Here's the drawing with two shaded views (mm, measured from the low corner). I have some questions. A direction names the side the tool comes from. Coordinates: 2 decimals unless noted, no trailing zeros. Order: outer loops, then holes, each group sorted by start corner. A loop starts at its lowest first (then second) coordinate and runs counter-clockwise, first axis right, second up. Notation, with made-up numbers: (-21, -29.75) - (-4, -29.75) arc R31 ccw to (-4, 5.25) - close; hole circle Ø5 at (-34, 13.25). An arc over 180 degrees is marked (long way). Answer as a JSON object with one key per item and string values. Group by question number.
(1) Imagine slicing it at D-D, the plane z = 10. Write out the boundary of the cut face in (x, y) (3 decimals), and give its area (3 significant figures).
(2) Will these pins go through, and if not, where does the flat tip stop? P1, Ø4, axis at x = 22, z = 3.5, coming from the -Y side; P2, Ø1, axis at y = 6, z = 2, coming from the -X side; P3, Ø1, axis at x = 29, z = 3, coming from the +Y side.
(3) Please list where these lines run through material, in increasing order: probe 1 along Y at (x, z) = (4, 3.5) (3 decimals); probe 2 along Z at (x, y) = (17.5, 2); probe 3 along X at (y, z) = (2.5, 9.25).
(4) We'd pull the mould along Y, two halves only. Please class the marked faces 1, 2, 3 and 4: pulls with the +Y half, pulls with the -Y half, needs draft (parallel to the pull), parting line crosses it, or undercut.
(5) Imagine slicing it at A-A, the plane x = 4. Write out the boundary of the cut face in (y, z) (3 decimals), and give its area (3 significant figures).
(6) Imagine slicing it at B-B, the plane y = 3. Write out the boundary of the cut face in (x, z).
(7) Imagine slicing it at C-C, the plane z = 2. Write out the boundary of the cut face in (x, y) (1 decimal), and give its area (3 significant figures).
(8) Which directions (+Z, -Z, +X, -X, +Y, -Y) give clear straight access to the entire face, cutting with the end or side of a thin tool? Please do the marked faces 5 and 6.
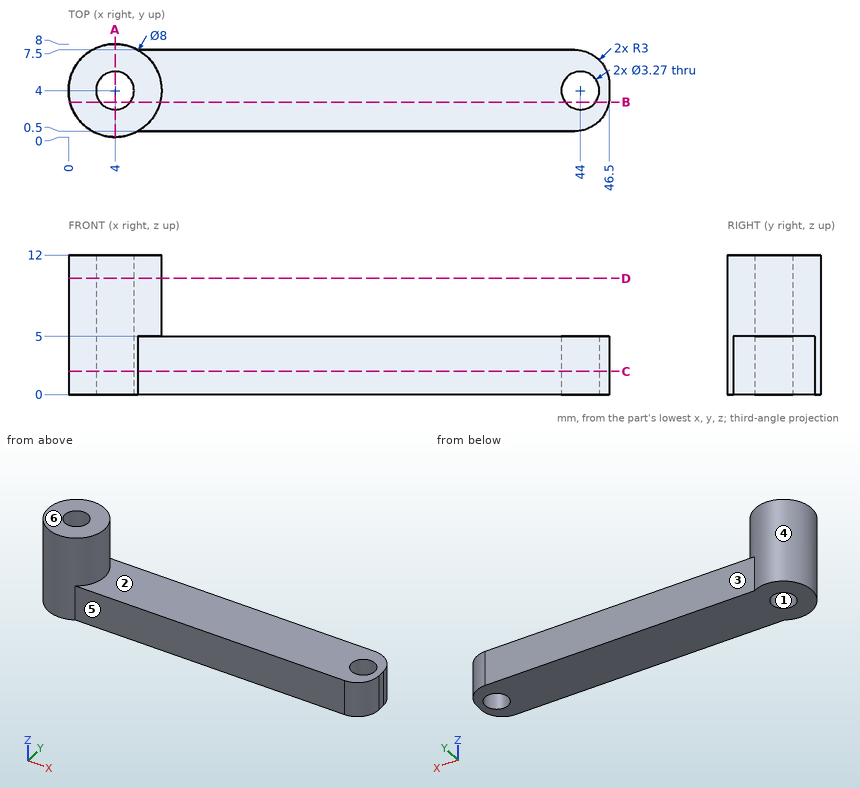
Result set:
{
 "1": {"outline": "circle Ø8 at (4, 4); hole circle Ø3.27 at (4, 4)", "area": "41.9 mm^2"},
 "2": {"P1": "stops at y = 0.5", "P2": "stops at x = 0.29", "P3": "stops at y = 7.5"},
 "3": {"probe 1": "y = 0 to 2.365, 5.635 to 8", "probe 2": "z = 0 to 5", "probe 3": "x = 0.29 to 3.35, 4.65 to 7.71"},
 "4": {"face 1": "undercut", "face 2": "needs draft", "face 3": "pulls with the +Y half", "face 4": "parting line crosses it"},
 "5": {"outline": "(0, 0) - (2.365, 0) - (2.365, 12) - (0, 12) - close; (5.635, 0) - (8, 0) - (8, 12) - (5.635, 12) - close", "area": "56.8 mm^2"},
 "6": {"outline": "(0.13, 0) - (2.71, 0) - (2.71, 12) - (0.13, 12) - close; (5.29, 0) - (42.71, 0) - (42.71, 5) - (7.87, 5) - (7.87, 12) - (5.29, 12) - close; (45.29, 0) - (46.46, 0) - (46.46, 5) - (45.29, 5) - close"},
 "7": {"outline": "(5.9, 0.5) - (43.5, 0.5) arc R3 ccw to (46.5, 3.5) - (46.5, 4.5) arc R3 ccw to (43.5, 7.5) - (5.9, 7.5) arc R4 ccw (long way) to start; hole circle Ø3.3 at (4, 4); hole circle Ø3.3 at (44, 4)", "area": "303 mm^2"},
 "8": {"face 5": "+Z, -Z, +X, -Y", "face 6": "+Z, +X, -X, +Y, -Y"}
}
